Verification items for the finished model (mm, model axes). Face numbers are marked on the shaded views. A direction names the side the tool comes from. Round coordinates to 2 decimals unless told otherwise and drop trailing zeros. Write each loop counter-clockwise with the first axis right and the second up, starting at its lowest first coordinate (ties: lowest second). Pieces come first, ordered by that corner, then holes.
from build123d import *

# Parameters (mm, degrees)
SKETCH_1_R          = 1.4
EXTRUDE_1_DEPTH     = 1.5
FILLET_1_R          = 5
EXTRUDE_2_DEPTH     = 0.5
CUT_EXTRUDE_1_DEPTH = 2.5
SKETCH_3_W          = 51.26
SKETCH_3_H          = 5.2
CUT_EXTRUDE_2_DEPTH = 2.5
CUT_EXTRUDE_3_DEPTH = 2.5
SKETCH_5_R          = 1.5
CUT_EXTRUDE_4_DEPTH = 2.5
CUT_EXTRUDE_5_DEPTH = 0.3
CHAMFER_1_SIZE      = 0.2
CUT_EXTRUDE_6_DEPTH = 2


with BuildPart() as part:
    # 草图1 → 凸台-拉伸1 (new body)
    with BuildSketch(Plane(origin=(0, 0, 0), x_dir=(1, 0, 0), z_dir=(0, 1, 0))):
        with BuildLine():
            Line((3, 0), (67.5, 0))
            ThreePointArc((67.5, 0), (72.621320344, -2.121320344), (70.5, 3))
            Line((70.5, 3), (70.5, 31))
            ThreePointArc((70.5, 31), (72.621320344, 36.121320344), (67.5, 34))
            Line((67.5, 34), (3, 34))
            ThreePointArc((3, 34), (-2.121320344, 36.121320344), (0, 31))
            Line((0, 31), (0, 3))
            ThreePointArc((0, 3), (-2.121320344, -2.121320344), (3, 0))
        make_face()
        with Locations(Location((0, 0, 0), (0, 0, 270))):
            Circle(SKETCH_1_R, mode=Mode.SUBTRACT)
        with Locations(Location((70.5, 0, 0), (0, 0, 270))):
            Circle(SKETCH_1_R, mode=Mode.SUBTRACT)
        with Locations(Location((70.5, 34, 0), (0, 0, 270))):
            Circle(SKETCH_1_R, mode=Mode.SUBTRACT)
        with Locations(Location((0, 34, 0), (0, 0, 270))):
            Circle(SKETCH_1_R, mode=Mode.SUBTRACT)
    extrude(amount=EXTRUDE_1_DEPTH)

    # 圆角1
    fillet_1_edges = [part.edges().sort_by_distance(p)[0] for p in [
        (70.5, 0.75, -31),
        (70.5, 0.75, -3),
        (67.5, 0.75, 0),
        (3, 0.75, 0),
        (0, 0.75, -3),
        (0, 0.75, -31),
        (3, 0.75, -34),
        (67.5, 0.75, -34),
    ]]
    fillet(fillet_1_edges, radius=FILLET_1_R)

    # 草图9 → 凸台-拉伸2 (add)
    with BuildSketch(Plane.XZ):
        with BuildLine():
            Line((3.2, -4.5), (3.2, -29.5))
            ThreePointArc((3.2, -29.5), (4.020101013, -31.479898987), (6, -32.3))
            Line((6, -32.3), (66, -32.3))
            ThreePointArc((66, -32.3), (67.979898987, -31.479898987), (68.8, -29.5))
            Line((68.8, -29.5), (68.8, -4.5))
            ThreePointArc((68.8, -4.5), (67.979898987, -2.520101013), (66, -1.7))
            Line((66, -1.7), (6, -1.7))
            ThreePointArc((6, -1.7), (4.020101013, -2.520101013), (3.2, -4.5))
        make_face()
    extrude(amount=EXTRUDE_2_DEPTH)

    # 草图2 → 切除-拉伸1 (cut)
    with BuildSketch(Plane(origin=(0, 1.5, 0), x_dir=(1, 0, 0), z_dir=(0, 1, 0))):
        with BuildLine():
            Line((48.45, 9.95), (34.15, 9.95))
            ThreePointArc((34.15, 9.95), (34.079289322, 9.979289322), (34.05, 10.05))
            Line((34.05, 10.05), (34.05, 24.35))
            ThreePointArc((34.05, 24.35), (34.079289322, 24.420710678), (34.15, 24.45))
            Line((34.15, 24.45), (48.45, 24.45))
            ThreePointArc((48.45, 24.45), (48.520710678, 24.420710678), (48.55, 24.35))
            Line((48.55, 24.35), (48.55, 10.05))
            ThreePointArc((48.55, 10.05), (48.520710678, 9.979289322), (48.45, 9.95))
        make_face()
    extrude(amount=-CUT_EXTRUDE_1_DEPTH, mode=Mode.SUBTRACT)

    # 草图3 → 切除-拉伸2 (cut)
    with BuildSketch(Plane(origin=(0, 1.5, 0), x_dir=(1, 0, 0), z_dir=(0, 1, 0))):
        with Locations((36, 28.5)):
            Rectangle(SKETCH_3_W, SKETCH_3_H)
    extrude(amount=-CUT_EXTRUDE_2_DEPTH, mode=Mode.SUBTRACT)

    # 草图4 → 切除-拉伸3 (cut)
    with BuildSketch(Plane(origin=(0, 1.5, 0), x_dir=(1, 0, 0), z_dir=(0, 1, 0))):
        with BuildLine():
            Line((48.7, 7.1), (53.7, 7.1))
            ThreePointArc((53.7, 7.1), (53.770710678, 7.070710678), (53.8, 7))
            Line((53.8, 7), (53.8, 2.1))
            ThreePointArc((53.8, 2.1), (53.770710678, 2.029289322), (53.7, 2))
            Line((53.7, 2), (48.7, 2))
            ThreePointArc((48.7, 2), (48.629289322, 2.029289322), (48.6, 2.1))
            Line((48.6, 2.1), (48.6, 7))
            ThreePointArc((48.6, 7), (48.629289322, 7.070710678), (48.7, 7.1))
        make_face()
    extrude(amount=-CUT_EXTRUDE_3_DEPTH, mode=Mode.SUBTRACT)

    # 草图5 → 切除-拉伸4 (cut)
    with BuildSketch(Plane(origin=(0, 1.5, 0), x_dir=(1, 0, 0), z_dir=(0, 1, 0))):
        with Locations(Location((34.98, 5.09, 0), (0, 0, 270))):
            Circle(SKETCH_5_R)
        with Locations(Location((38.54, 5.09, 0), (0, 0, 270))):
            Circle(SKETCH_5_R)
    extrude(amount=-CUT_EXTRUDE_4_DEPTH, mode=Mode.SUBTRACT)

    # 草图7 → 切除-拉伸5 (cut)
    with BuildSketch(Plane(origin=(0, 1.5, 0), x_dir=(1, 0, 0), z_dir=(0, 1, 0))):
        with BuildLine():
            Line((43.10725502, 6.55256053), (43.098194404, 5.868627045))
            Line((43.098194404, 5.868627045), (44.440296605, 6.84))
            Line((44.440296605, 6.84), (43.123465549, 7.776199492))
            Line((43.123465549, 7.776199492), (43.114019957, 7.063206413))
            ThreePointArc((43.114019957, 7.063206413), (42.146572001, 3.56478636), (45.440296605, 5.09))
            ThreePointArc((45.440296605, 5.09), (45.190296605, 5.34), (44.940296605, 5.09))
            ThreePointArc((44.940296605, 5.09), (42.504765307, 3.917489365), (43.10725502, 6.55256053))
        make_face()
        with BuildLine():
            Line((29.833898496, 4.717073646), (29.833898496, 7.938528917))
            ThreePointArc((29.833898496, 7.938528917), (30.083898496, 8.188528917), (30.333898496, 7.938528917))
            Line((30.333898496, 7.938528917), (30.333898496, 4.717073646))
            ThreePointArc((30.333898496, 4.717073646), (30.083898496, 4.467073646), (29.833898496, 4.717073646))
        make_face()
        with BuildLine():
            ThreePointArc((29.235650456, 6.901208233), (30.08487931, 3.09000024), (30.930369668, 6.902039336))
            ThreePointArc((30.930369668, 6.902039336), (30.598055855, 6.781343315), (30.718751875, 6.449029502))
            ThreePointArc((30.718751875, 6.449029502), (30.084634106, 3.59000018), (29.447712466, 6.448406175))
            ThreePointArc((29.447712466, 6.448406175), (29.56808249, 6.780838209), (29.235650456, 6.901208233))
        make_face()
    extrude(amount=-CUT_EXTRUDE_5_DEPTH, mode=Mode.SUBTRACT)

    # 倒角1
    chamfer_1_edges = [part.edges().sort_by_distance(p)[0] for p in [
        (70.5, 0, -1.4),
        (72.621320344, 1.5, 2.121320344),
        (35.25, 1.5, 0),
        (-2.121320344, 1.5, 2.121320344),
        (0, 1.5, -17),
        (-2.121320344, 1.5, -36.121320344),
        (35.25, 1.5, -34),
        (72.621320344, 1.5, -36.121320344),
        (70.5, 1.5, -17),
        (66.420065511, 1.5, 0.493060906),
        (4.079934489, 1.5, 0.493060906),
        (-0.493060906, 1.5, -4.079934489),
        (-0.493060906, 1.5, -29.920065511),
        (4.079934489, 1.5, -34.493060906),
        (66.420065511, 1.5, -34.493060906),
        (70.993060906, 1.5, -29.920065511),
        (70.993060906, 1.5, -4.079934489),
    ]]
    chamfer(chamfer_1_edges, length=CHAMFER_1_SIZE)

    # 草图10 → 切除-拉伸6 (cut)
    with BuildSketch(Plane(origin=(0, 1.5, 0), x_dir=(1, 0, 0), z_dir=(0, 1, 0))):
        with BuildLine():
            Line((3.7, 9.4), (11.3, 9.4))
            ThreePointArc((11.3, 9.4), (11.441421356, 9.458578644), (11.5, 9.6))
            Line((11.5, 9.6), (11.5, 11.8))
            ThreePointArc((11.5, 11.8), (11.441421356, 11.941421356), (11.3, 12))
            Line((11.3, 12), (3.7, 12))
            ThreePointArc((3.7, 12), (3.558578644, 11.941421356), (3.5, 11.8))
            Line((3.5, 11.8), (3.5, 9.6))
            ThreePointArc((3.5, 9.6), (3.558578644, 9.458578644), (3.7, 9.4))
        make_face()
    extrude(amount=-CUT_EXTRUDE_6_DEPTH, mode=Mode.SUBTRACT)


solid = part.part
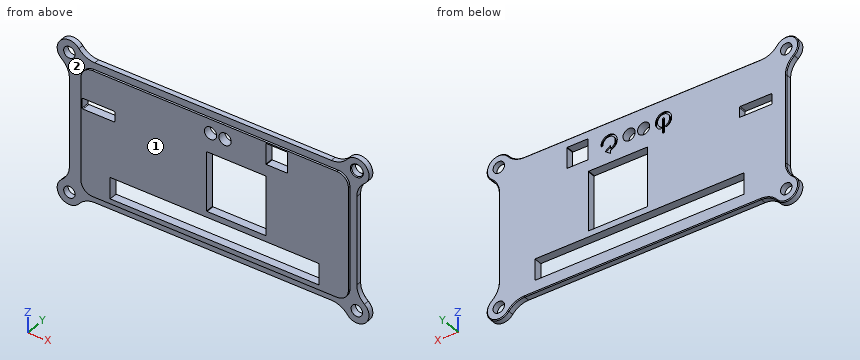
Q1. Depth check by flat-ended pin: P1, Ø3, axis at x = 0, z = -34, coming from the -Y side; P2, Ø0.6, axis at y = 0.5, z = -19, coming from the +X side; P3, Ø0.6, axis at y = 0.5, z = -5, coming from the -X side. Enter the tip coordinate at first touch or a pass-through.
Recorded:
P1: stops at y = 0
P2: stops at x = 70.5
P3: stops at x = -0.24
Q2. Sectioned sample at A-A (x = 38.54). Enter the section's corners in (y, z).
Recorded:
outline: (-0.5, -32.3) - (0, -32.3) - (0, -34) - (1.3, -34) - (1.5, -33.8) - (1.5, -31.1) - (-0.5, -31.1) - close; (-0.5, -25.9) - (1.5, -25.9) - (1.5, -24.45) - (-0.5, -24.45) - close; (-0.5, -9.95) - (1.5, -9.95) - (1.5, -6.59) - (-0.5, -6.59) - close; (-0.5, -3.59) - (1.5, -3.59) - (1.5, -0.2) - (1.3, 0) - (0, 0) - (0, -1.7) - (-0.5, -1.7) - close
Q3. Material ranges on line 1 along Z through (x, y) = (10.5, 0.5); line 2 along X through (y, z) = (0.5, -10); line 3 along Z through (x, y) = (38.5, 1.4), recorded low to high.
Recorded:
line 1: z = -34 to -31.1, -25.9 to -12, -9.4 to 0
line 2: x = 0 to 3.5, 11.5 to 34.06, 48.54 to 70.5
line 3: z = -33.9 to -31.1, -25.9 to -24.45, -9.95 to -6.59, -3.59 to -0.1
Q4. Sectioned sample at C-C (x = 50). Enter the section's corners in (y, z).
Recorded:
outline: (-0.5, -32.3) - (0, -32.3) - (0, -34) - (1.3, -34) - (1.5, -33.8) - (1.5, -31.1) - (-0.5, -31.1) - close; (-0.5, -25.9) - (1.5, -25.9) - (1.5, -7.1) - (-0.5, -7.1) - close; (-0.5, -2) - (1.5, -2) - (1.5, -0.2) - (1.3, 0) - (0, 0) - (0, -1.7) - (-0.5, -1.7) - close
Q5. Sectioned sample at B-B (z = -27). Enter the section's corners in (x, y), plus the area to 3 significant figures.
Recorded:
outline: (0, 0) - (3.2, 0) - (3.2, -0.5) - (10.37, -0.5) - (10.37, 1.5) - (0.2, 1.5) - (0, 1.3) - close; (61.63, -0.5) - (68.8, -0.5) - (68.8, 0) - (70.5, 0) - (70.5, 1.3) - (70.3, 1.5) - (61.63, 1.5) - close
area: 36.0 mm2
Q6. Sectioned sample at D-D (x = 25). Enter the section's corners in (y, z), plus the area to 3 significant figures.
Recorded:
outline: (-0.5, -32.3) - (0, -32.3) - (0, -34) - (1.3, -34) - (1.5, -33.8) - (1.5, -31.1) - (-0.5, -31.1) - close; (-0.5, -25.9) - (1.5, -25.9) - (1.5, -0.2) - (1.3, 0) - (0, 0) - (0, -1.7) - (-0.5, -1.7) - close
area: 55.9 mm2
Q7. Tool access check on the marked faces 1 and 2. Record the directions out of +Z, -Z, +X, -X, +Y, -Y that give a thin tool (end or side, any length) a straight path to the whole face; none if there is none.
Recorded:
face 1: +Z, -Z, +X, -X, -Y
face 2: -Y
